Here's how the part is built. I have some questions about the finished solid (model axes, mm). Face numbers are marked on the shaded views. A direction names the side the tool comes from. Round coordinates to 2 decimals unless told otherwise and drop trailing zeros. Write each loop counter-clockwise with the first axis right and the second up, starting at its lowest first coordinate (ties: lowest second). Pieces come first, ordered by that corner, then holes. Notation, with made-up numbers: (-39, -26.5) -> (18, -26.5) arc R5 ccw to (18, -18.5) -> close; hole circle Ø4 at (-26.5, -36). An arc over 180 degrees is marked (long way). Answer in a Markdown table with one row per item. Add a question column.
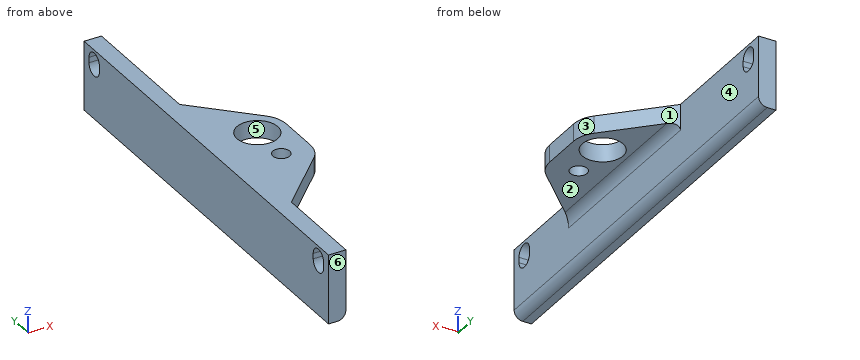
from build123d import *

# Parameters (mm, degrees)
BOSS_EXTRUDE1_DEPTH = 6.35
SKETCH2_R           = 7.475
SKETCH2_R_2         = 3.0999938
BOSS_EXTRUDE2_DEPTH = 6.35
FILLET1_R           = 3.175


with BuildPart() as part:
    # Sketch1 → Boss-Extrude1 (new body)
    with BuildSketch(Plane(origin=(0, 0, 0), x_dir=(0, 0, -1), z_dir=(1, 0, 0))):
        Polygon((-4.34721, -76.524739), (4.34721, -76.524739), (21.05279, -76.524739), (21.05279, 76.524739), (4.34721, 76.524739), (-4.34721, 76.524739), align=None)
        with BuildLine():
            Line((0, 73.438639), (2, 73.438639))
            ThreePointArc((2, 73.438639), (5.2639, 70.174739), (2, 66.910839))
            Line((2, 66.910839), (0, 66.910839))
            ThreePointArc((0, 66.910839), (-3.2639, 70.174739), (0, 73.438639))
        make_face(mode=Mode.SUBTRACT)
        with BuildLine():
            Line((0, -66.910839), (2, -66.910839))
            ThreePointArc((2, -66.910839), (5.2639, -70.174739), (2, -73.438639))
            Line((2, -73.438639), (0, -73.438639))
            ThreePointArc((0, -73.438639), (-3.2639, -70.174739), (0, -66.910839))
        make_face(mode=Mode.SUBTRACT)
    extrude(amount=BOSS_EXTRUDE1_DEPTH)

    # Sketch2 → Boss-Extrude2 (add)
    with BuildSketch(Plane.XY.offset(4.34721)):
        with BuildLine():
            Line((6.35, 27.567699439), (26.28122122, 7.63647822))
            ThreePointArc((26.28122122, 7.63647822), (28.589851021, 4.181369555), (29.400534, 0.105791))
            Line((29.400534, 0.105791), (29.400534, -14.894209))
            ThreePointArc((29.400534, -14.894209), (28.589851021, -18.969787555), (26.28122122, -22.42489622))
            Line((26.28122122, -22.42489622), (6.35, -42.356117439))
            Line((6.35, -42.356117439), (6.35, 27.567699439))
        make_face()
        with Locations((18.750534, 0.105791)):
            Circle(SKETCH2_R, mode=Mode.SUBTRACT)
        with Locations((18.750534, -14.894209)):
            Circle(SKETCH2_R_2, mode=Mode.SUBTRACT)
    extrude(amount=-BOSS_EXTRUDE2_DEPTH)

    # Fillet1
    fillet1_edges = [part.edges().sort_by_distance(p)[0] for p in [
        (6.35, 0, -21.05279),
        (6.35, -7.394209, -2.00279),
    ]]
    fillet(fillet1_edges, radius=FILLET1_R)


solid = part.part
Item 1: If we section it at B-B on y = -26.5: Please give me the cut outline in (x, z) (3 decimals).
Item 2: If we section it at D-D on x = 8: Please give me the cut outline in (y, z), then the cut area to 3 significant figures.
Item 3: I need wall thicknesses on line 1 along Y through (x, z) = (5, -0.5); line 2 along X through (y, z) = (9.5, -12.25); line 3 along Y through (x, z) = (22.5, -1.25). Which ranges of each line are inside material? Lowest first, please. Write a range as from..to.
Item 4: If we mould it in two halves opening along Y, with no side actions, what happens to the marked faces 3, 4, 5 and 6? For each: pulls with the +Y half, pulls with the -Y half, needs draft (parallel to the pull), parting line crosses it, or undercut.
Item 5: If we section it at A-A on y = 5: Please give me the cut outline in (x, z) (3 decimals).
Item 6: On a 3-axis mill with a long thin cutter (end or side, diameter ignored), from which of +Z, -Z, +X, -X, +Y, -Y can I reach the whole of each face in a straight line? I mean the marked faces 1 and 2. Say none if no direction works.
Item 7: If we section it at C-C on z = -9: Please give me the cut outline in (x, y), then the cut area to 3 significant figures.
Item 8: For P1, Ø1.5, axis at y = 37.5, z = -1, coming from the +X side; P2, Ø6, axis at y = 16, z = -15, coming from the +X side; P3, Ø5.5, axis at x = 18.75, y = -14.89, coming from the -Z side; P4, Ø6, axis at x = 20.5, y = 6.5, coming from the -Z side, each with a flat end and sliding along its axis, tell me the tip position at first contact or that it passes through.
Results list:
| question | item | result |
|---|---|---|
| 1 | outline | (0, -21.053) -> (3.175, -21.053) arc R3.175 ccw to (6.35, -17.878) -> (6.35, -5.178) arc R3.175 cw to (9.525, -2.003) -> (22.206, -2.003) -> (22.206, 4.347) -> (0, 4.347) -> close |
| 2 | outline | (-40.71, -2.39) -> (25.92, -2.39) -> (25.92, 4.35) -> (-40.71, 4.35) -> close |
| 2 | area | 449 mm² |
| 3 | line 1 | -76.52..-73.44, -66.91..66.91, 73.44..76.52 |
| 3 | line 2 | 0..6.35 |
| 3 | line 3 | -26.21..-6.36, 6.57..11.42 |
| 4 | face 3 | pulls with the +Y half |
| 4 | face 4 | needs draft |
| 4 | face 5 | undercut |
| 4 | face 6 | pulls with the -Y half |
| 5 | outline | (0, -21.053) -> (3.175, -21.053) arc R3.175 ccw to (6.35, -17.878) -> (6.35, -5.178) arc R3.175 cw to (9.525, -2.003) -> (13.101, -2.003) -> (13.101, 4.347) -> (0, 4.347) -> close; (24.401, -2.003) -> (28.209, -2.003) -> (28.209, 4.347) -> (24.401, 4.347) -> close |
| 6 | face 1 | +Z, -Z, +X, +Y |
| 6 | face 2 | -Z, +X, +Y, -Y |
| 7 | outline | (0, -76.52) -> (6.35, -76.52) -> (6.35, 76.52) -> (0, 76.52) -> close |
| 7 | area | 972 mm² |
| 8 | P1 | x = 6.35 |
| 8 | P2 | x = 6.35 |
| 8 | P3 | through |
| 8 | P4 | z = -2 |
